Source: CAD feature listing. Evaluate the final solid. Frame: model axes, mm. Coordinates: 2 decimals unless noted, no trailing zeros. Order: outer loops, then holes, each group sorted by start corner. A loop starts at its lowest first (then second) coordinate and runs counter-clockwise, first axis right, second up.
```python
from build123d import *

# Parameters (mm, degrees)
SKETCH1_R           = 3.81
BOSS_EXTRUDE1_DEPTH = 2
BOSS_EXTRUDE2_DEPTH = 2
FILLET1_R           = 0.254
SKETCH3_R           = 0.75
CUT_EXTRUDE1_DEPTH  = 2
SKETCH4_R           = 1.5
CUT_EXTRUDE2_DEPTH  = 3


with BuildPart() as part:
    # Sketch1 → Boss-Extrude1 (new body)
    with BuildSketch(Plane(origin=(0, 0, 0), x_dir=(1, 0, 0), z_dir=(0, 1, 0))):
        Circle(SKETCH1_R)
    extrude(amount=BOSS_EXTRUDE1_DEPTH)

    # Sketch2 → Boss-Extrude2 (add)
    with BuildSketch(Plane(origin=(0, 2, 0), x_dir=(1, 0, 0), z_dir=(0, 1, 0))):
        with BuildLine():
            Line((0, -13.5), (3.247846855, -1.991881223))
            ThreePointArc((3.247846855, -1.991881223), (0, -3.81), (-3.247846855, -1.991881223))
            Line((-3.247846855, -1.991881223), (0, -13.5))
        make_face()
        with BuildLine():
            ThreePointArc((-3.247846855, 1.991881223), (0, 3.81), (3.247846855, 1.991881223))
            Line((3.247846855, 1.991881223), (0, 13.5))
            Line((0, 13.5), (-3.247846855, 1.991881223))
        make_face()
    extrude(amount=-BOSS_EXTRUDE2_DEPTH)

    # Fillet1
    fillet1_edges = [part.edges().sort_by_distance(p)[0] for p in [
        (0, 1, -13.5),
        (0, 1, 13.5),
    ]]
    fillet(fillet1_edges, radius=FILLET1_R)

    # Sketch3 → Cut-Extrude1 (cut)
    with BuildSketch(Plane(origin=(0, 2, 0), x_dir=(1, 0, 0), z_dir=(0, 1, 0))):
        with Locations((0, 8.5)):
            Circle(SKETCH3_R)
        with Locations((0, -8.5)):
            Circle(SKETCH3_R)
    extrude(amount=-CUT_EXTRUDE1_DEPTH, mode=Mode.SUBTRACT)

    # Sketch4 → Cut-Extrude2 (cut, through all)
    with BuildSketch(Plane.XZ):
        Circle(SKETCH4_R)
    extrude(amount=-CUT_EXTRUDE2_DEPTH, mode=Mode.SUBTRACT)


solid = part.part
```
Q1. Pin query (flat end, axial travel): P1, Ø1, axis at y = 1.5, z = -8, coming from the -X side; P2, Ø1, axis at y = 1.5, z = -9.5, coming from the -X side. Return the tip coordinate at first contact, or that it passes through.
Solutions:
P1: stops at x = -1.69
P2: stops at x = -1.27
Q2. Section query D-D on x = 1.25. Output: boundary loops of the cut face in (y, z), plus the area to 3 significant figures.
Solutions:
outline: (0, -9.07) - (2, -9.07) - (2, -0.83) - (0, -0.83) - close; (0, 0.83) - (2, 0.83) - (2, 9.07) - (0, 9.07) - close
area: 33.0 mm2
Q3. Material intervals for line 1 along Z through (x, y) = (0, 0.9); line 2 along X through (y, z) = (0.3, -0.75); line 3 along X through (y, z) = (1.5, -8.5), sorted ascending.
Solutions:
line 1: z = -12.82 to -9.25, -7.75 to -1.5, 1.5 to 7.75, 9.25 to 12.82
line 2: x = -3.74 to -1.3, 1.3 to 3.74
line 3: x = -1.41 to -0.75, 0.75 to 1.41
Q4. Section query A-A on x = 0. Output: boundary loops of the cut face in (y, z), plus the area to 3 significant figures.
Solutions:
outline: (0, -12.82) - (2, -12.82) - (2, -9.25) - (0, -9.25) - close; (0, -7.75) - (2, -7.75) - (2, -1.5) - (0, -1.5) - close; (0, 1.5) - (2, 1.5) - (2, 7.75) - (0, 7.75) - close; (0, 9.25) - (2, 9.25) - (2, 12.82) - (0, 12.82) - close
area: 39.3 mm2
Q5. Section query B-B on z = 0. Output: boundary loops of the cut face in (x, y).
Solutions:
outline: (-3.81, 0) - (-1.5, 0) - (-1.5, 2) - (-3.81, 2) - close; (1.5, 0) - (3.81, 0) - (3.81, 2) - (1.5, 2) - close
Q6. Section query C-C on y = 0.6. Output: boundary loops of the cut face in (x, z).
Solutions:
outline: (-3.25, -1.99) - (-0.24, -12.63) arc R0.25 ccw to (0.24, -12.63) - (3.25, -1.99) arc R3.81 ccw to (3.25, 1.99) - (0.24, 12.63) arc R0.25 ccw to (-0.24, 12.63) - (-3.25, 1.99) arc R3.81 ccw to start; hole circle Ø3 at (0, 0); hole circle Ø1.5 at (0, -8.5); hole circle Ø1.5 at (0, 8.5)
